For this review, take the finished solid that the model builds, in its own axes (mm). Face numbers are marked on the shaded views. A direction names the side the tool comes from. Give positions to 0.01 mm unless a question says otherwise; leave off trailing zeros. Write each loop counter-clockwise with the first axis right and the second up, starting at its lowest first coordinate (ties: lowest second). Pieces come first, ordered by that corner, then holes. Notation, with made-up numbers: M 17,37.25 L 51,37.25 A28 ccw 51,59.25 Z; hole C 69.5,84 d9. An arc over 180 degrees is marked long. One line per item, written item: value. Start each with the question number.
Item 1: Clearance check with flat-ended pins moving along their axes: pin 1 Ø1 at (x, z) = (-5, -10) entering from -Y; pin 2 Ø4 at (x, z) = (-5, 20.5) entering from +Y; pin 3 Ø1.5 at (x, z) = (-6, 3) entering from -Y. State where each tip first meets the part, or that it passes through.
Item 2: Consider section A-A, the plane x = 0. Write out the cut boundary in (y, z), and give its area (3 significant figures).
Item 3: Consider section D-D, the plane z = 47. Write out the cut boundary in (x, y).
Item 4: Tool access review of the marked faces 1, 2 and 3: name each direction out of +Z, -Z, +X, -X, +Y, -Y from which nothing blocks a thin tool from reaching the whole face with its end or side.
Item 5: To check wall thickness, follow probe 1 along X at (y, z) = (0.5, 31); probe 2 along Z at (x, y) = (4.25, -5.5); probe 3 along X at (y, z) = (4.5, -1). State the ranges of each line that lie inside material, in increasing order.
Item 6: Consider section C-C, the plane z = 22.5. Write out the cut boundary in (x, y), and give its area (3 significant figures).
```python
from build123d import *

# Parameters (mm, degrees)
ESQUISSE1_R          = 8
BASE_EXTRUSION_DEPTH = 44
ESQUISSE2_R          = 5
BOSS_EXTRU_1_DEPTH   = 9
ESQUISSE3_R          = 6
BOSS_EXTRU_2_DEPTH   = 20
CHANFREIN1_SIZE      = 1


with BuildPart() as part:
    # Esquisse1 → Base-Extrusion (new body)
    with BuildSketch(Plane.XY):
        Circle(ESQUISSE1_R)
    extrude(amount=BASE_EXTRUSION_DEPTH)

    # Esquisse2 → Boss.-Extru.1 (add)
    with BuildSketch(Plane.XY.offset(44)):
        Circle(ESQUISSE2_R)
    extrude(amount=BOSS_EXTRU_1_DEPTH)

    # Esquisse3 → Boss.-Extru.2 (add)
    with BuildSketch(Plane(origin=(0, 0, 0), x_dir=(-1, 0, 0), z_dir=(0, 0, -1))):
        with Locations(Location((0, 0, 0), (0, 0, 180))):
            Circle(ESQUISSE3_R)
    extrude(amount=BOSS_EXTRU_2_DEPTH)

    # Chanfrein1
    chanfrein1_edges = [part.edges().sort_by_distance(p)[0] for p in [
        (-6, 0, -20),
    ]]
    chamfer(chanfrein1_edges, length=CHANFREIN1_SIZE)


solid = part.part
```
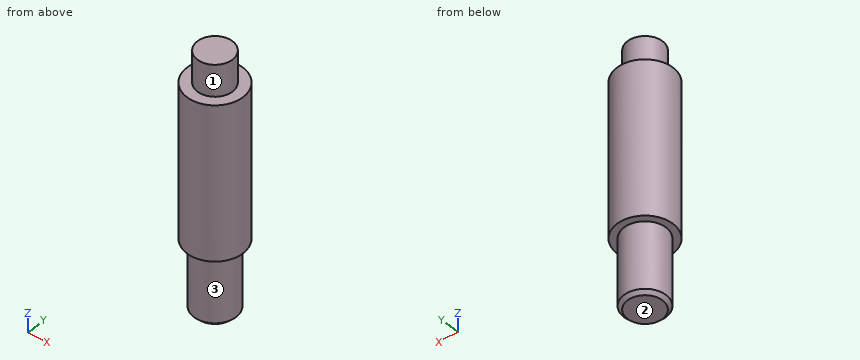
Model answer:
1. pin 1: stops at y = -3.97
1. pin 2: stops at y = 7.42
1. pin 3: stops at y = -6.04
2. outline: M -8,0 L -6,0 L -6,-19 L -5,-20 L 5,-20 L 6,-19 L 6,0 L 8,0 L 8,44 L 5,44 L 5,53 L -5,53 L -5,44 L -8,44 Z
2. area: 1,030 mm2
3. outline: C 0,0 d10
4. face 1: +Z
4. face 2: -Z, +X, -X, +Y, -Y
4. face 3: -Z
5. probe 1: x = -7.98 to 7.98
5. probe 2: z = 0 to 44
5. probe 3: x = -3.97 to 3.97
6. outline: C 0,0 d16
6. area: 201 mm2
